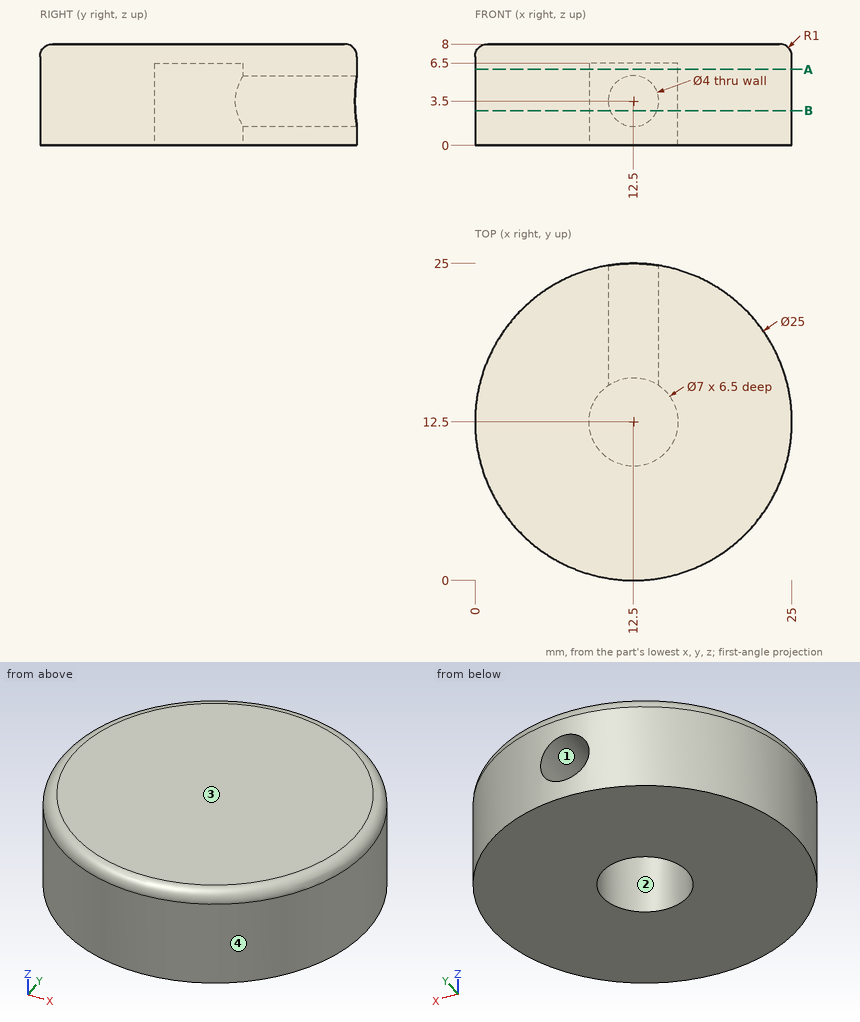
Verification items for this drawing (mm, ordinates from the low corner). Coordinates: 2 decimals unless noted, no trailing zeros. Order: outer loops, then holes, each group sorted by start corner. A loop starts at its lowest first (then second) coordinate and runs counter-clockwise, first axis right, second up. Notation, with made-up numbers: (0, 2.5) - (40, 2.5) arc R28 cw to (40, 35.5) - close; hole circle Ø11 at (83.25, 0.25). An arc over 180 degrees is marked (long way). Answer in a Markdown table with one row per item. Add a question column.
1. Draft check along X on the marked faces 1, 2, 3 and 4. Enter one of: +X half, -X half, draft (parallel to the pull), parting line (faces both ways), or undercut.
2. Section check A-A (z = 6). Enter the section's corners in (x, y), plus the area to 3 significant figures.
3. Material ranges on L1, parallel to Y at x = 14.75, z = 5; L2, parallel to Z at x = 10.5, y = 13.5; L3, parallel to X at y = 20.75, z = 7.5, recorded low to high. Write a range as [from, to].
4. Gauge pin test, flat ends, axial feed: pin 1 Ø3 at (y, z) = (16, 3.5) entering from -X; pin 2 Ø3 at (y, z) = (3.5, 3.5) entering from -X; pin 3 Ø3.5 at (x, y) = (11.5, 12) entering from -Z. Record the tip position at first contact, or that the pin passes through.
5. Section check B-B (z = 2.75). Enter the section's corners in (x, y), plus the area to 3 significant figures.
Data:
| question | item | result |
|---|---|---|
| 1 | face 1 | undercut |
| 1 | face 2 | undercut |
| 1 | face 3 | draft |
| 1 | face 4 | parting line |
| 2 | outline | circle Ø25 at (12.5, 12.5); hole circle Ø7 at (12.5, 12.5) |
| 2 | area | 452 mm² |
| 3 | L1 | y = [0.2, 9.82], [15.18, 24.8] |
| 3 | L2 | z = [6.5, 8] |
| 3 | L3 | x = [3.29, 21.71] |
| 4 | pin 1 | stops at x = 0.16 |
| 4 | pin 2 | stops at x = 2.5 |
| 4 | pin 3 | stops at z = 6.5 |
| 5 | outline | (10.65, 15.47) - (10.65, 24.86) arc R12.5 ccw (long way) to (14.35, 24.86) - (14.35, 15.47) arc R3.5 cw (long way) to start |
| 5 | area | 419 mm² |
